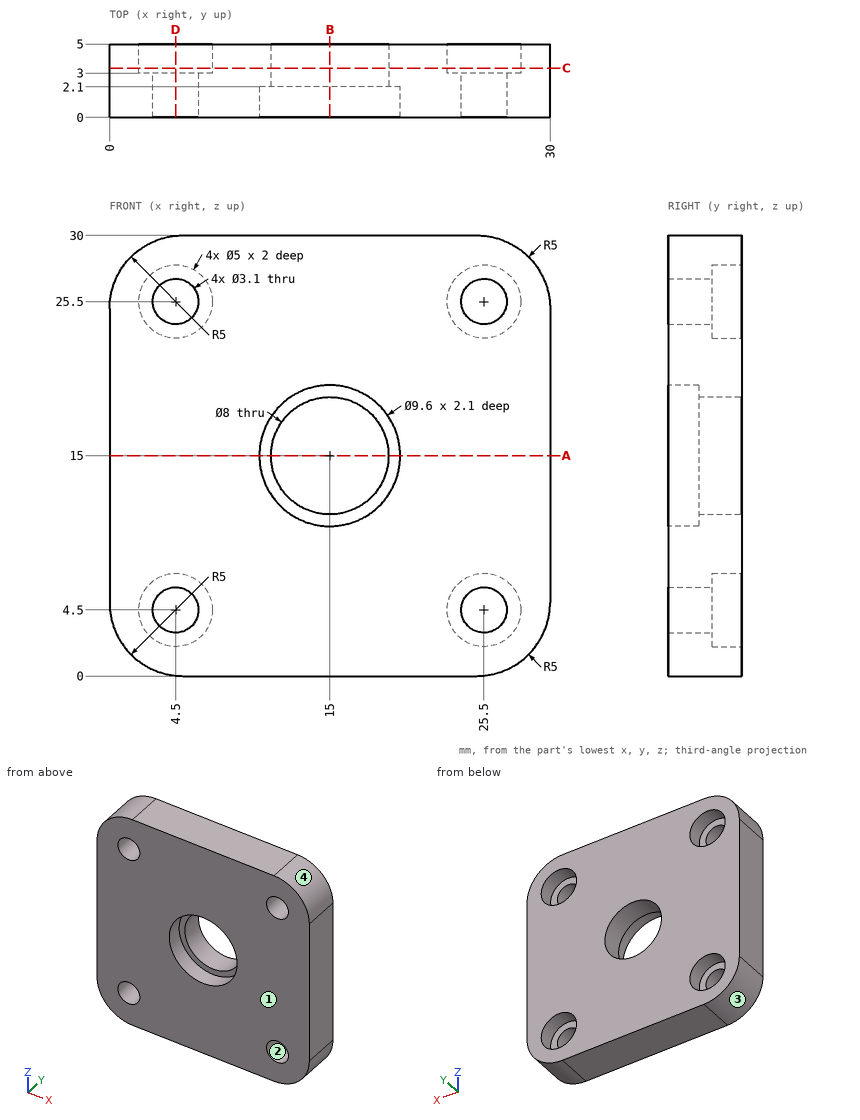
Job drawing, mm, ordinate dimensions from the low corner. One solid piece. Coordinates: 2 decimals unless noted, no trailing zeros. Loops run counter-clockwise (first coordinate to the right, second up) from the corner with the lowest first, then second, coordinate; pieces in that order, holes last. Notation, with made-up numbers: (-15, -37.75) - (1, -37.75) arc R32 ccw to (1, -1.75) - close; hole circle Ø1 at (12.25, -5.75). An arc over 180 degrees is marked (long way). Answer as a JSON object with one key per item and string values. Group by question number.
(1) Flat gauge pins, fed straight in: pin 1 (2.5 mm diameter, centred on x = 5, z = 25.5, fed in from +Y); pin 2 (3 mm diameter, centred on x = 25.5, z = 4.5, fed in from -Y); pin 3 (1 mm diameter, centred on y = 2.5, z = 4, fed in from +X); pin 4 (1 mm diameter, centred on x = 12.5, z = 18, fed in from -Y). Where does each tip first touch, or does it go through?
(2) Probe line 1 along Z through (x, y) = (15, 0.5); line 2 along Z through (x, y) = (4.5, 4); line 3 along Z through (x, y) = (3, 4.6). List the from-to ranges inside material, lowest first.
(3) Cut at B-B (x = 15). Give the cut face in (y, z), then the cut area to 3 significant figures.
(4) Cut at C-C (y = 3.35). Give the cut face in (x, z).
(5) Two-plate mould, pull along X, no slides. Class the marked faces 1, 2, 3 and 4: released by +X, released by -X, zero draft, split by the parting line, or undercut.
(6) Cut at A-A (z = 15). Give the cut face in (x, y), then the cut area to 3 significant figures.
(7) Cut at D-D (x = 4.5). Give the cut face in (y, z).
Geometry says:
{
 "1": {"pin 1": "stops at y = 3", "pin 2": "passes through", "pin 3": "stops at x = 29.97", "pin 4": "stops at y = 2.1"},
 "2": {"line 1": "z = 0 to 10.2, 19.8 to 30", "line 2": "z = 0.03 to 2, 7 to 23, 28 to 29.97", "line 3": "z = 0.42 to 2.5, 6.5 to 23.5, 27.5 to 29.58"},
 "3": {"outline": "(0, 0) - (5, 0) - (5, 11) - (2.1, 11) - (2.1, 10.2) - (0, 10.2) - close; (0, 19.8) - (2.1, 19.8) - (2.1, 19) - (5, 19) - (5, 30) - (0, 30) - close", "area": "107 mm^2"},
 "4": {"outline": "(0, 5) arc R5 ccw to (5, 0) - (25, 0) arc R5 ccw to (30, 5) - (30, 25) arc R5 ccw to (25, 30) - (5, 30) arc R5 ccw to (0, 25) - close; hole circle Ø5 at (4.5, 4.5); hole circle Ø5 at (4.5, 25.5); hole circle Ø8 at (15, 15); hole circle Ø5 at (25.5, 4.5); hole circle Ø5 at (25.5, 25.5)"},
 "5": {"face 1": "zero draft", "face 2": "undercut", "face 3": "released by -X", "face 4": "released by +X"},
 "6": {"outline": "(0, 0) - (10.2, 0) - (10.2, 2.1) - (11, 2.1) - (11, 5) - (0, 5) - close; (19, 2.1) - (19.8, 2.1) - (19.8, 0) - (30, 0) - (30, 5) - (19, 5) - close", "area": "107 mm^2"},
 "7": {"outline": "(0, 0.03) - (5, 0.03) - (5, 2) - (3, 2) - (3, 2.95) - (0, 2.95) - close; (0, 6.05) - (3, 6.05) - (3, 7) - (5, 7) - (5, 23) - (3, 23) - (3, 23.95) - (0, 23.95) - close; (0, 27.05) - (3, 27.05) - (3, 28) - (5, 28) - (5, 29.97) - (0, 29.97) - close"}
}
